```python
from build123d import *

# Parameters (mm, degrees)
F1_R     = 29
F1_R_2   = 27
F2_DEPTH = 68.948
F3_R     = 29
F3_R_2   = 25
F3_R_3   = 23
F4_DEPTH = 2
F5_DEPTH = 8.284


with BuildPart() as f2:
    # F1 (on face) → F2 (new body)
    with BuildSketch(Plane.XY):
        Circle(F1_R)
        Circle(F1_R_2, mode=Mode.SUBTRACT)
    extrude(amount=F2_DEPTH)

    # F3 (on face) → F4 (join)
    with BuildSketch(Plane(origin=(0, 0, 0), x_dir=(1, 0, 0), z_dir=(0, 0, -1))):
        Circle(F3_R)
        Circle(F3_R_2, mode=Mode.SUBTRACT)
        Circle(F3_R_2)
        Circle(F3_R_3, mode=Mode.SUBTRACT)
    extrude(amount=F4_DEPTH)

    # F3 (on face) → F5 (join)
    with BuildSketch(Plane(origin=(0, 0, 0), x_dir=(1, 0, 0), z_dir=(0, 0, -1))):
        Circle(F3_R)
        Circle(F3_R_2, mode=Mode.SUBTRACT)
    extrude(amount=-F5_DEPTH)


solid = f2.part
```
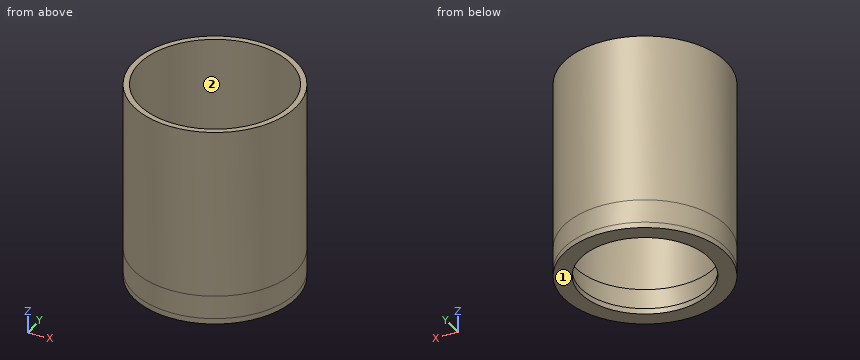
Design review of the part built by this model. Coordinates are the model's own, in mm. Face numbers are marked on the shaded views. Coordinates: 2 decimals unless noted, no trailing zeros. Order: outer loops, then holes, each group sorted by start corner. A loop starts at its lowest first (then second) coordinate and runs counter-clockwise, first axis right, second up.
1) Take a section at C-C, the plane z = 37. Give the boundary of the cut face in (x, y).
2) Wall thickness on line 1 along X through (y, z) = (0, -0.5); line 2 along Y through (x, z) = (1, 10); line 3 along X through (y, z) = (0, 57): over which ranges is each line inside the solid? List them lowest first.
3) Clearance check with flat-ended pins moving along their axes: pin 1 (1 mm diameter, centred on y = -12, z = 39.5, fed in from -X); pin 2 (6 mm diameter, centred on y = -18.5, z = 48, fed in from +X); pin 3 (1 mm diameter, centred on x = -16.5, z = 59, fed in from +Y). State where each tip first meets the part, or that it passes through.
4) Mouldability with a two-part tool opening along Y and no side actions: class the marked faces 1 and 2 as +Y half, -Y half, draft (parallel to the pull), parting line (faces both ways), or undercut.
5) Take a section at B-B, the plane x = -12. Give the boundary of the cut face in (y, z).
6) Take a section at D-D, the plane x = -24. Give the boundary of the cut face in (y, z), and give its area (3 significant figures).
7) Take a section at A-A, the plane y = 0. Give the boundary of the cut face in (x, z), and give its area (3 significant figures).
Returned:
1. outline: circle Ø58 at (0, 0); hole circle Ø54 at (0, 0)
2. line 1: x = -29 to -23, 23 to 29
2. line 2: y = -28.98 to -26.98, 26.98 to 28.98
2. line 3: x = -29 to -27, 27 to 29
3. pin 1: stops at x = -26.62
3. pin 2: stops at x = 24.51
3. pin 3: stops at y = 24.19
4. face 1: draft
4. face 2: undercut
5. outline: (-26.4, -2) - (-19.62, -2) - (-19.62, 0) - (-21.93, 0) - (-21.93, 8.28) - (-24.19, 8.28) - (-24.19, 68.95) - (-26.4, 68.95) - close; (19.62, -2) - (26.4, -2) - (26.4, 68.95) - (24.19, 68.95) - (24.19, 8.28) - (21.93, 8.28) - (21.93, 0) - (19.62, 0) - close
6. outline: (-16.28, -2) - (16.28, -2) - (16.28, 68.95) - (12.37, 68.95) - (12.37, 8.28) - (7, 8.28) - (7, 0) - (-7, 0) - (-7, 8.28) - (-12.37, 8.28) - (-12.37, 68.95) - (-16.28, 68.95) - close
6. area: 693 mm2
7. outline: (-29, -2) - (-23, -2) - (-23, 0) - (-25, 0) - (-25, 8.28) - (-27, 8.28) - (-27, 68.95) - (-29, 68.95) - close; (23, -2) - (29, -2) - (29, 68.95) - (27, 68.95) - (27, 8.28) - (25, 8.28) - (25, 0) - (23, 0) - close
7. area: 333 mm2
